CAD build for the part. Positions are in the model's coordinates, mm. Face numbers are marked on the shaded views. A direction names the side the tool comes from. Round coordinates to 2 decimals unless told otherwise and drop trailing zeros. Loops run counter-clockwise (first coordinate to the right, second up) from the corner with the lowest first, then second, coordinate; pieces in that order, holes last. Notation, with made-up numbers: M -12,70 L 33,70 A30 cw 33,104 Z; hole C 13,-36 d3. An arc over 180 degrees is marked long. Use one line per item in the form item = value.
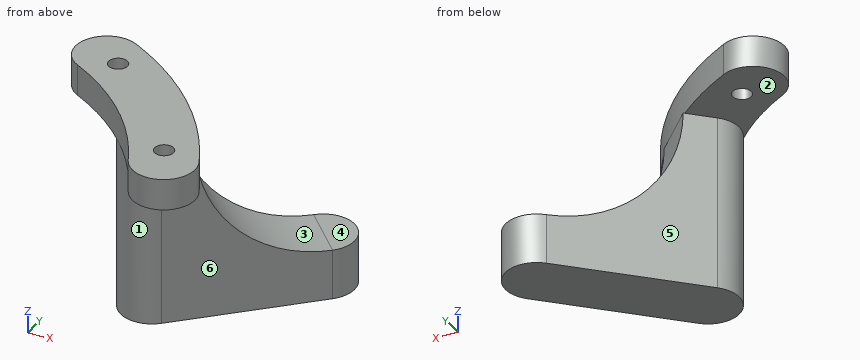
from build123d import *

# Parameters (mm, degrees)
SKETCH014_R             = 1.5
PAD007_DEPTH            = 5
SKETCH015_R             = 5
PAD008_DEPTH            = 33
PAD009_DEPTH            = 5
PAD010_DEPTH            = 8
BODY004_PLACEMENT_ANGLE = 45


with BuildPart() as part:
    # Sketch014 → Pad007 (new body)
    with BuildSketch(Plane.XY):
        with BuildLine():
            ThreePointArc((49.280643, -16.595729), (52, 9e-06), (49.280638, 16.595745))
            ThreePointArc((49.280638, 16.595745), (42.946367, 19.738522), (39.803594, 13.404249))
            ThreePointArc((39.803592, -13.404255), (42, -3e-06), (39.803594, 13.404249))
            ThreePointArc((39.803592, -13.404255), (42.946378, -19.738526), (49.280643, -16.595729))
        make_face()
        with Locations((45.398514, 12.164495)):
            Circle(SKETCH014_R, mode=Mode.SUBTRACT)
        with Locations((45.398514, -12.164495)):
            Circle(SKETCH014_R, mode=Mode.SUBTRACT)
    extrude(amount=-PAD007_DEPTH)

    # Sketch015 → Pad008 (join)
    with BuildSketch(Plane.XY):
        with Locations((47, 0)):
            Circle(SKETCH015_R)
    extrude(amount=-PAD008_DEPTH)

    # Sketch016 → Pad009 (join, symmetric)
    with BuildSketch(Plane.XZ):
        with BuildLine():
            Line((47, -5), (47, -33))
            Line((47, -33), (72, -33))
            Line((72, -33), (72, -25))
            ThreePointArc((52, -5), (57.857864, -19.142136), (72, -25))
            Line((52, -5), (47, -5))
        make_face()
    extrude(amount=PAD009_DEPTH, both=True)

    # Sketch017 → Pad010 (join)
    with BuildSketch(Plane.XY.offset(-33)):
        with BuildLine():
            ThreePointArc((72, -5), (77, 0), (72, 5))
            Line((72, 5), (72, -5))
        make_face()
    extrude(amount=PAD010_DEPTH)


with BuildPart() as part_1:
    # Body004 placement: moved
    add(part.part.moved(Location((0, 0, 23))).rotate(Axis((0, 0, 23), (0, 0, 1)), BODY004_PLACEMENT_ANGLE))


solid = part_1.part
1. Cut at B-B on x = 20.5. Write the cut outline in (y, z).
Completed:
outline = M 36.66,18 L 47.09,18 L 47.09,23 L 36.66,23 Z
2. Probe line 1 along X through (y, z) = (42, 18.5); line 2 along X through (y, z) = (23.5, 19.6); line 3 along Y through (x, z) = (23, 19). List the from-to ranges inside material, lowest first. Write a range as from..to.
Completed:
line_1 = 15.89..22.75, 24.25..30.66
line_2 = 34.81..39.2, 42.2..46.39
line_3 = 35.14..39.29, 42.12..46.64
3. Pull direction Z, two halves, no side cores. Call the marked faces 1, 2 and 3: +Z half, -Z half, draft (parallel to the pull), parting line (faces both ways), or undercut.
Completed:
face_1 = draft
face_2 = -Z half
face_3 = +Z half
4. Drop flat-ended pins along their axis: P1, Ø19, axis at x = 38.5, y = 27.5, coming from the -Z side; P2, Ø1, axis at x = 38, z = -0.5, coming from the -Y side; P3, Ø8, axis at x = 23, z = 15, coming from the -Y side; P4, Ø6, axis at y = 37, z = 1, coming from the -X side. Give the stop position or say it passes through.
Completed:
P1 = -10
P2 = 30.43
P3 = 33.26
P4 = 28.29
5. Tool access for the marked faces 4, 5 and 6: list every direction of +Z, -Z, +X, -X, +Y, -Y with a clear straight run to the whole face (end or side of a thin tool).
Completed:
face_4 = +Z, +X, +Y
face_5 = -Z, -X, +Y
face_6 = -Z, +X, -Y
